from build123d import *

# Parameters (mm, degrees)
SKETCH1_R                = 14.325
SKETCH1_R_2              = 13.825
BOSS_EXTRUDE1_DEPTH      = 10
SKETCH2_R                = 14.325
SKETCH3_R                = 12.165
SKETCH5_R                = 1.51
BOSS_EXTRUDE3_DEPTH      = 21.11
BOSS_EXTRUDE3_DEPTH_BACK = 17.23
SKETCH6_W                = 1
SKETCH6_H                = 4.34
CUT_EXTRUDE1_DEPTH       = 15.3250001
CUT_EXTRUDE1_DEPTH_BACK  = 15.3250001


with BuildPart() as part:
    # Sketch1 → Boss-Extrude1 (new body)
    with BuildSketch(Plane.XY):
        Circle(SKETCH1_R)
        Circle(SKETCH1_R_2, mode=Mode.SUBTRACT)
    extrude(amount=BOSS_EXTRUDE1_DEPTH)

    # Sketch2 → Loft1 section 0
    with BuildSketch(Plane.XY.offset(10)):
        Circle(SKETCH2_R)
    # Sketch3 → Loft1 section 1
    with BuildSketch(Plane.XY.offset(11.92)):
        Circle(SKETCH3_R)
    loft()

    # Sketch5 → Boss-Extrude3 (add, two sides)
    with BuildSketch(Plane.XY.offset(11.92)) as boss_extrude3_sk:
        Circle(SKETCH5_R)
    extrude(amount=BOSS_EXTRUDE3_DEPTH)
    extrude(boss_extrude3_sk.sketch, amount=-BOSS_EXTRUDE3_DEPTH_BACK)

    # Sketch6 → Cut-Extrude1 (cut, two sides)
    with BuildSketch(Plane(origin=(0, 0, 0), x_dir=(1, 0, 0), z_dir=(0, 1, 0))) as cut_extrude1_sk:
        with Locations((-1.78, -18.09)):
            Rectangle(SKETCH6_W, SKETCH6_H)
        with Locations((1.78, -18.09)):
            Rectangle(SKETCH6_W, SKETCH6_H)
    extrude(amount=CUT_EXTRUDE1_DEPTH, mode=Mode.SUBTRACT)
    extrude(cut_extrude1_sk.sketch, amount=-CUT_EXTRUDE1_DEPTH_BACK, mode=Mode.SUBTRACT)


solid = part.part
Source: CAD feature listing. Evaluate the final solid. Frame: model axes, mm. A direction names the side the tool comes from. Give positions to 0.01 mm unless a question says otherwise; leave off trailing zeros. Write each loop counter-clockwise with the first axis right and the second up, starting at its lowest first coordinate (ties: lowest second). Pieces come first, ordered by that corner, then holes. Notation, with made-up numbers: M 8,26 L 26,26 A19 cw 26,58 Z; hole C 20,39.5 d9. An arc over 180 degrees is marked long. Return JSON: item names as keys, results as strings. Group by question number.
1) Material intervals for line 1 along Y through (x, z) = (0, 5.5) (3 decimals); line 2 along Z through (x, y) = (3.75, -10); line 3 along Y through (x, z) = (12.25, 3.5), sorted ascending. Write a range as [from, to].
2) Cut plane A-A, the plane z = 1.5. Output: boundary loops of the cut face in (x, y) (3 decimals).
3) Set-up query: faces 4 (the face through (1.28, 0, 18)), 5 (the face through (-1.28, 0, 18)), 6 (the face through (13.187, 4.153, 4.93)), 7 (the face through (-1.51, 0.07, 22.33)). Return all of +Z, -Z, +X, -X, +Y, -Y with unobstructed straight access to the full face (end or side cutting, diameter ignored); none if empty.
4) Cut plane B-B, the plane x = 0. Output: boundary loops of the cut face in (y, z) (3 decimals), plus the area to 3 significant figures.
5) Cut plane C-C, the plane z = 19.5. Output: boundary loops of the cut face in (x, y).
6) Pull-direction query (X, two-part tool) for faces 1 (the face through (0, 0, -5.31)), 2 (the face through (13.663, 4.303, 4.93)), 3 (the face through (3, 0, 10)); classes: pulls with the +X half, pulls with the -X half, needs draft (parallel to the pull), parting line crosses it, or undercut.
7) Pin query (flat end, axial travel): P1, Ø5, axis at y = 5.5, z = -1.5, coming from the -X side; P2, Ø10, axis at y = 5.5, z = -1, coming from the -X side; P3, Ø7.5, axis at x = 6, y = 0, coming from the +Z side. Return the tip coordinate at first contact, or that it passes through.
Recorded:
{
 "1": {"line 1": "y = [-14.325, -13.825], [-1.51, 1.51], [13.825, 14.325]", "line 2": "z = [10, 11.92]", "line 3": "y = [-7.43, -6.41], [6.41, 7.43]"},
 "2": {"outline": "C 0,0 d28.65; C 0,0 d3.02; hole C 0,0 d27.65"},
 "3": {"face 4": "+X, +Y, -Y", "face 5": "-X, +Y, -Y", "face 6": "-Z", "face 7": "+Z"},
 "4": {"outline": "M -14.325,0 L -13.825,0 L -13.825,10 L -1.51,10 L -1.51,-5.31 L 1.51,-5.31 L 1.51,10 L 13.825,10 L 13.825,0 L 14.325,0 L 14.325,10 L 12.165,11.92 L 1.51,11.92 L 1.51,33.03 L -1.51,33.03 L -1.51,11.92 L -12.165,11.92 L -14.325,10 Z", "area": "171 mm²"},
 "5": {"outline": "M -1.28,-0.8 A1.51 ccw 1.28,-0.8 L 1.28,0.8 A1.51 ccw -1.28,0.8 Z"},
 "6": {"face 1": "needs draft", "face 2": "parting line crosses it", "face 3": "undercut"},
 "7": {"P1": "stops at x = -13.89", "P2": "stops at x = -14.31", "P3": "stops at z = 11.92"}
}
